The listing builds one solid part. Answer for the finished solid, in the listing's coordinates (mm). A direction names the side the tool comes from. Coordinates: 2 decimals unless noted, no trailing zeros. Loops run counter-clockwise (first coordinate to the right, second up) from the corner with the lowest first, then second, coordinate; pieces in that order, holes last. Notation, with made-up numbers: M 71.25,54.25 L 110.25,54.25 A16 cw 110.25,69.25 Z; hole C 12.5,-22 d10. An arc over 180 degrees is marked long. Answer as a JSON object with one key per item and string values. Group by question number.
1. A cutting plane is placed at C-C on x = -14.5. Give the vertices of the cut face in (y, z).
2. Determine the mould class of faces 3 (the face through (0, 0, 12)), 4 (the face through (-18.063, 16.245, 11.979)), 5 (the face through (-8.6, 3.07, 11.98)) for opening direction X: released by +X, released by -X, zero draft, split by the parting line, or undercut.
3. A cutting plane is placed at D-D on z = 11.05. State how many separate pieces and enclosed holes the cut face has, and give its area (3 significant figures).
4. Given pin 1 (0.9 mm diameter, centred on y = 7, z = 12, fed in from -X); pin 2 (3 mm diameter, centred on x = -7.5, y = 19.5, fed in from +Z), each flat-ended and moving along its own axis, determine where each tip first touches the part or whether it passes through.
5. For faces 1 (the face through (-11, 8, 12)), 2 (the face through (9.5, 0.5, 12)), determine the directions among +Z, -Z, +X, -X, +Y, -Y from which every point of the face is accessible in a straight line to the end or side of a thin tool.
6. A cutting plane is placed at B-B on y = 18.5. Give the vertices of the cut face in (x, z), and give its area (3 significant figures).
7. A cutting plane is placed at A-A on x = -6.5. Give the vertices of the cut face in (y, z), and give its area (3 significant figures).
8. Straight lines are drawn through the part: L1, parallel to X at y = 8.5, z = 12.3; L2, parallel to Y at x = -7, z = 12.45; L3, parallel to X at y = 5.5, z = 12.7. For each, find the intervals that lie inside material, in ascending order.
from build123d import *

# Parameters (mm, degrees)
SKETCH081_R     = 1.6
PAD046_DEPTH    = 3
CHAMFER026_SIZE = 1
FILLET021_R     = 3


with BuildPart() as part:
    # Sketch081 → Pad046 (new body)
    with BuildSketch(Plane.XY):
        Polygon((10, 55), (-25, 55), (-25, 17.468578), (-11, 15), (-11, 0), (10, 0), align=None)
        with Locations((-7.5, 19.5)):
            Circle(SKETCH081_R, mode=Mode.SUBTRACT)
        with Locations((7.5, 19.5)):
            Circle(SKETCH081_R, mode=Mode.SUBTRACT)
        with Locations((7.5, 9.5)):
            Circle(SKETCH081_R, mode=Mode.SUBTRACT)
        with Locations((-7.5, 9.5)):
            Circle(SKETCH081_R, mode=Mode.SUBTRACT)
        with Locations((-7, 52)):
            Circle(SKETCH081_R, mode=Mode.SUBTRACT)
        with Locations((6, 52)):
            Circle(SKETCH081_R, mode=Mode.SUBTRACT)
        with Locations((-7, 3)):
            Circle(SKETCH081_R, mode=Mode.SUBTRACT)
        with Locations((6, 3)):
            Circle(SKETCH081_R, mode=Mode.SUBTRACT)
        with Locations((-13.75, 19.5)):
            Circle(SKETCH081_R, mode=Mode.SUBTRACT)
    extrude(amount=PAD046_DEPTH)

    # Chamfer026
    chamfer026_edges = [part.edges().sort_by_distance(p)[0] for p in [
        (10, 0, 1.5),
        (10, 55, 1.5),
        (-25, 55, 1.5),
    ]]
    chamfer(chamfer026_edges, length=CHAMFER026_SIZE)

    # Fillet021
    fillet021_edges = [part.edges().sort_by_distance(p)[0] for p in [
        (-25, 17.468578, 1.5),
        (-11, 15, 1.5),
        (-11, 0, 1.5),
    ]]
    fillet(fillet021_edges, radius=FILLET021_R)


with BuildPart() as part_1:
    # Body038 placement: moved
    add(part.part.moved(Location((-2e-06, -1.5e-05, 10.499998))))


solid = part_1.part
From the geometry:
{
 "1": {"outline": "M 15.62,10.5 L 18.09,10.5 L 18.09,13.5 L 15.62,13.5 Z; M 20.91,10.5 L 55,10.5 L 55,13.5 L 20.91,13.5 Z"},
 "2": {"face 3": "zero draft", "face 4": "released by -X", "face 5": "undercut"},
 "3": {"separate pieces": "1", "enclosed holes": "9", "area": "1,620 mm²"},
 "4": {"pin 1": "stops at x = -11", "pin 2": "passes through"},
 "5": {"face 1": "+Z, -Z, -X, -Y", "face 2": "+Z, -Z, +X, -Y"},
 "6": {"outline": "M -24.61,10.5 L -15,10.5 L -15,13.5 L -24.61,13.5 Z; M -12.5,10.5 L -8.75,10.5 L -8.75,13.5 L -12.5,13.5 Z; M -6.25,10.5 L 6.25,10.5 L 6.25,13.5 L -6.25,13.5 Z; M 8.75,10.5 L 10,10.5 L 10,13.5 L 8.75,13.5 Z", "area": "81.3 mm²"},
 "7": {"outline": "M 0,10.5 L 1.48,10.5 L 1.48,13.5 L 0,13.5 Z; M 4.52,10.5 L 8.25,10.5 L 8.25,13.5 L 4.52,13.5 Z; M 10.75,10.5 L 18.25,10.5 L 18.25,13.5 L 10.75,13.5 Z; M 20.75,10.5 L 50.48,10.5 L 50.48,13.5 L 20.75,13.5 Z; M 53.52,10.5 L 55,10.5 L 55,13.5 L 53.52,13.5 Z", "area": "132 mm²"},
 "8": {"L1": "x = -11 to -8.75, -6.25 to 6.25, 8.75 to 10", "L2": "y = 0 to 1.4, 4.6 to 7.98, 11.02 to 17.98, 21.02 to 50.4, 53.6 to 55", "L3": "x = -11 to 10"}
}
